Work out the finished part from the listing and answer in its coordinate system (mm). Round coordinates to 2 decimals unless told otherwise and drop trailing zeros. Write each loop counter-clockwise with the first axis right and the second up, starting at its lowest first coordinate (ties: lowest second). Pieces come first, ordered by that corner, then holes. Notation, with made-up numbers: (3, -2.75) -> (9, -2.75) arc R28 cw to (9, 26.25) -> close; hole circle Ø3 at (52, -40). An arc over 180 degrees is marked (long way). Answer as a JSON object with one key per item and string values. Group by question number.
from build123d import *

# Parameters (mm, degrees)
F0_R     = 50.8
F1_DEPTH = 2.54
F3_DEPTH = 12.7
F5_DEPTH = 25.4
F7_DEPTH = 25.4
F9_DEPTH = 25.4


# Not quite as in the source:
# - a feature names something its author has since deleted; it is built from what else it names


with BuildPart() as f1:
    # F0 (on Top) → F1 (new body)
    with BuildSketch(Plane.XY):
        Circle(F0_R)
    extrude(amount=F1_DEPTH)

    # F2 (on face) → F3 (join)
    with BuildSketch(Plane.XY.offset(2.54)):
        Polygon((-50.8, 6.35), (-50.8, 0), (-50.8, -6.35), (-44.45, -6.35), (-44.45, 6.35), align=None)
        Polygon((16.725738686, -41.6698291982), (19.900738686, -47.1690905122), (30.899261314, -40.8190905122), (27.724261314, -35.3198291982), align=None)
        Polygon((27.724261314, 35.3198291982), (30.899261314, 40.8190905122), (19.900738686, 47.1690905122), (16.725738686, 41.6698291982), align=None)
    extrude(amount=F3_DEPTH)

    # F4 (on face) → F5 (cut)
    with BuildSketch(Plane.XZ.offset(6.35)):
        Polygon((-50.8, 15.24), (-50.8, 2.54), (-46.2367217033, 5.962595906), (-44.45, 7.3026908967), (-44.45, 15.24), align=None)
    extrude(amount=-F5_DEPTH, mode=Mode.SUBTRACT)

    # F6 (on face) → F7 (cut)
    with BuildSketch(Plane(origin=(5.499261314, 3.175, 0), x_dir=(-0.5, 0.8660254038, 0), z_dir=(0.8660254038, 0.5, 0))):
        Polygon((-50.0320994455, 6.7267423959), (-44.45, 2.54), (-44.45, 15.24), (-50.8, 15.24), (-50.8, 7.3026908967), align=None)
    extrude(amount=-F7_DEPTH, mode=Mode.SUBTRACT)

    # F8 (on face) → F9 (cut)
    with BuildSketch(Plane(origin=(-5.499261314, 3.175, 0), x_dir=(-0.5, -0.8660254038, 0), z_dir=(-0.8660254038, 0.5, 0))):
        Polygon((-50.8, 15.24), (-50.8, 7.3026908967), (-49.8044750842, 6.556017282), (-44.45, 2.54), (-44.45, 15.24), align=None)
    extrude(amount=-F9_DEPTH, mode=Mode.SUBTRACT)


solid = f1.part
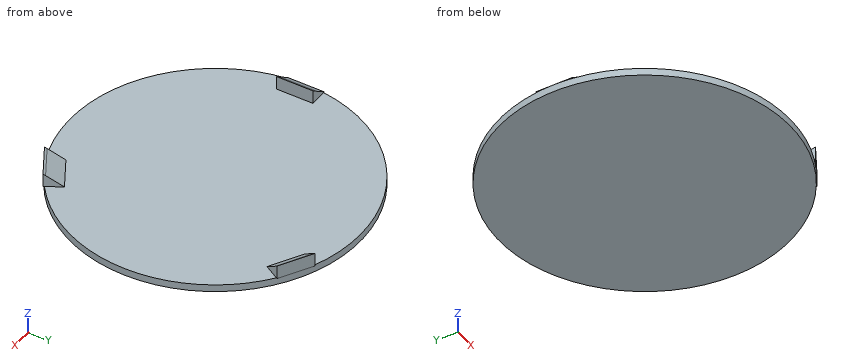
1) A cutting plane is placed at C-C on x = 0. Determine the outline of the cut face in (y, z), plus the area to 3 significant figures.
2) Each of these flat-tipped pins is pushed along its axis until it touches: P1, Ø1.5, axis at x = -2, y = -18.5, coming from the +Z side; P2, Ø2.5, axis at x = -47.5, z = 6, coming from the -Y side; P3, Ø1.4, axis at x = -48, z = 5, coming from the +Y side. Where does it stop, or does it pass through?
3) A cutting plane is placed at A-A on z = 4. Determine the outline of the cut face in (x, y), plus the area to 3 significant figures.
4) A cutting plane is placed at B-B on y = -4. Determine the outline of the cut face in (x, z), plus the area to 3 significant figures.
5) A cutting plane is placed at D-D on x = 14. Determine the outline of the cut face in (y, z), plus the area to 3 significant figures.
6) Straight lines are drawn through the part: L1, parallel to Z at x = 33.5, y = -11; L2, parallel to X at y = 13, z = 2.25; L3, parallel to Y at x = 21, z = 6.25. For each, find the intervals that lie inside material, in ascending order.
Established:
{
 "1": {"outline": "(-50.8, 0) -> (50.8, 0) -> (50.8, 2.54) -> (-50.8, 2.54) -> close", "area": "258 mm²"},
 "2": {"P1": "stops at z = 2.54", "P2": "stops at y = -6.35", "P3": "stops at y = 6.35"},
 "3": {"outline": "(-48.85, -6.35) -> (-44.45, -6.35) -> (-44.45, 6.35) -> (-48.85, 6.35) -> close; (17.7, -43.36) -> (19.9, -47.17) -> (30.9, -40.82) -> (28.7, -37.01) -> close; (17.7, 43.36) -> (28.7, 37.01) -> (30.9, 40.82) -> (19.9, 47.17) -> close", "area": "168 mm²"},
 "4": {"outline": "(-50.8, 2.54) -> (-50.64, 2.54) -> (-50.64, 0) -> (50.64, 0) -> (50.64, 2.54) -> (-44.45, 2.54) -> (-44.45, 7.3) -> close", "area": "272 mm²"},
 "5": {"outline": "(-48.83, 0) -> (48.83, 0) -> (48.83, 2.54) -> (-48.83, 2.54) -> close", "area": "248 mm²"},
 "6": {"L1": "z = 0 to 2.54", "L2": "x = -49.11 to 49.11", "L3": "y = -46.53 to -44.91, 44.91 to 46.53"}
}
